```python
from build123d import *

# Parameters (mm, degrees)
F2_R     = 11.176
F2_R_2   = 3.302
F3_DEPTH = 12.7
F4_SIZE  = 5.08


with BuildPart() as f1:
    # F0 (on Right) → F1 (revolve)
    with BuildSketch(Plane.YZ):
        Polygon((23.495, 21.188779), (3.302, 21.188779), (3.302, -16.767403), (6.35, -16.911221), align=None)
        Polygon((6.35, -16.911221), (3.302, -16.767403), (3.302, -23.261221), (6.35, -23.261221), align=None)
        Polygon((3.302, -23.261221), (3.302, -16.767403), (0, -16.6116), (0, -23.261221), align=None)
    revolve(axis=Axis((0, 0, 4.724398), (0, 0, -1)))

    # F2 (on face) → F3 (cut)
    with BuildSketch(Plane.XY.offset(21.188779)):
        Circle(F2_R)
        Circle(F2_R_2, mode=Mode.SUBTRACT)
    extrude(amount=-F3_DEPTH, mode=Mode.SUBTRACT)

    # F4
    f4_edges = [f1.edges().sort_by_distance(p)[0] for p in [
        (0, -23.495, 21.188779),
    ]]
    chamfer(f4_edges, length=F4_SIZE)


solid = f1.part
```
Verification items for the finished model (mm, model axes). A direction names the side the tool comes from. Coordinates: 2 decimals unless noted, no trailing zeros. Loops run counter-clockwise (first coordinate to the right, second up) from the corner with the lowest first, then second, coordinate; pieces in that order, holes last. Notation, with made-up numbers: (89.25, -6.5) - (111.25, -6.5) arc R27 cw to (111.25, 11.5) - close; hole circle Ø8 at (43.25, 35). An arc over 180 degrees is marked (long way). Return JSON: item names as keys, results as strings.
1. Tool access check on faces 1 (the flat face through (2, 3, 8.489)), 2 (the cylindrical face through (-6.2, -1.38, -20.04)), 3 (the flat face through (0, 0, -23.261)). Record the directions out of +Z, -Z, +X, -X, +Y, -Y that give a thin tool (end or side, any length) a straight path to the whole face; none if there is none.
Established:
{"face 1": "+Z", "face 2": "-Z", "face 3": "-Z, +X, -X, +Y, -Y"}
2. Thickness scan on L1, parallel to Y at x = 0, z = 16; L2, parallel to Y at x = 0, z = 14.5; L3, parallel to X at y = 2, z = -0.5. Record the ranges inside material, lowest first.
Established:
{"L1": "y = -21.16 to -11.18, 11.18 to 21.16", "L2": "y = -20.49 to -11.18, 11.18 to 20.49", "L3": "x = -13.59 to -2.63, 2.63 to 13.59"}
3. Section check B-B, the plane z = -15. Record the boundary of the cut face in (x, y), then the cut area to 3 significant figures.
Established:
{"outline": "circle Ø14.42 at (0, 0); hole circle Ø6.6 at (0, 0)", "area": "129 mm2"}
4. Mould release check, pull along X, two halves, no side actions. Record for faces 4 (the flat face through (-12, 0, 21.189)), 5 (the conical face through (5.59, 17.74, 20.9)), 6 (the cylindrical face through (-8.87, -6.8, 14.93)): +X half, -X half, draft (parallel to the pull), parting line (faces both ways), or undercut.
Established:
{"face 4": "draft", "face 5": "parting line", "face 6": "undercut"}
5. Go/stop test with flat-tipped pins: pin 1 (2 mm diameter, centred on y = 2, z = 10.5, fed in from -X); pin 2 (6 mm diameter, centred on x = 7, z = -4, fed in from -Y); pin 3 (10 mm diameter, centred on y = 2, z = -3, fed in from +X). Record where each tip stops, or that it passes through.
Established:
{"pin 1": "stops at x = -19.04", "pin 2": "stops at y = -12.18", "pin 3": "stops at x = 14.78"}
6. Section check A-A, the plane z = -20. Record the boundary of the cut face in (x, y).
Established:
{"outline": "circle Ø12.7 at (0, 0)"}
7. Section check C-C, the plane z = 12. Record the boundary of the cut face in (x, y).
Established:
{"outline": "circle Ø38.72 at (0, 0); hole circle Ø22.35 at (0, 0)"}
